```python
from build123d import *

# Parameters (mm, degrees)
SKETCH1_R               = 35
BOSS_EXTRUDE1_DEPTH     = 25
SKETCH2_R               = 30
CUT_EXTRUDE1_DEPTH      = 20
SKETCH3_R               = 25
CUT_EXTRUDE2_DEPTH      = 20
SKETCH4_R               = 27
CUT_EXTRUDE3_DEPTH      = 2.5
SKETCH5_R               = 55.910187051
CUT_EXTRUDE4_DEPTH      = 10
CUT_EXTRUDE6_DEPTH      = 52.720402164
CUT_EXTRUDE6_DEPTH_BACK = 52.720402164
SKETCH7_R               = 3.175


with BuildPart() as part:
    # Sketch1 → Boss-Extrude1 (new body)
    with BuildSketch(Plane(origin=(0, 0, 0), x_dir=(1, 0, 0), z_dir=(0, 1, 0))):
        with Locations(Location((0, 0, 0), (0, 0, 270))):
            Circle(SKETCH1_R)
    extrude(amount=BOSS_EXTRUDE1_DEPTH)

    # Sketch2 → Cut-Extrude1 (cut)
    with BuildSketch(Plane(origin=(0, 25, 0), x_dir=(1, 0, 0), z_dir=(0, 1, 0))):
        with Locations(Location((0, 0, 0), (0, 0, 270))):
            Circle(SKETCH2_R)
    extrude(amount=-CUT_EXTRUDE1_DEPTH, mode=Mode.SUBTRACT)

    # Sketch3 → Cut-Extrude2 (cut)
    with BuildSketch(Plane.XZ):
        with Locations(Location((0, 0, 0), (0, 0, 270))):
            Circle(SKETCH3_R)
    extrude(amount=-CUT_EXTRUDE2_DEPTH, mode=Mode.SUBTRACT)

    # Sketch4 → Cut-Extrude3 (cut)
    with BuildSketch(Plane(origin=(0, 5, 0), x_dir=(1, 0, 0), z_dir=(0, 1, 0))):
        with Locations(Location((0, 0, 0), (0, 0, 270))):
            Circle(SKETCH4_R)
    extrude(amount=-CUT_EXTRUDE3_DEPTH, mode=Mode.SUBTRACT)

    # Sketch5 → Cut-Extrude4 (cut)
    with BuildSketch(Plane(origin=(0, 25, 0), x_dir=(1, 0, 0), z_dir=(0, 1, 0))):
        Circle(SKETCH5_R)
    extrude(amount=-CUT_EXTRUDE4_DEPTH, mode=Mode.SUBTRACT)

    # Sketch7 → Cut-Extrude6 (cut, two sides: drawn at the far end of the back side and taken through both)
    with BuildSketch(Plane.XY.offset(-CUT_EXTRUDE6_DEPTH_BACK)):
        with Locations((0, 9.572)):
            Circle(SKETCH7_R)
    extrude(amount=CUT_EXTRUDE6_DEPTH + CUT_EXTRUDE6_DEPTH_BACK, mode=Mode.SUBTRACT)


solid = part.part
```
Input: part model. Units: mm. Frame: model coordinates. A direction names the side the tool comes from. Give positions to 0.01 mm unless a question says otherwise; leave off trailing zeros. Loops run counter-clockwise (first coordinate to the right, second up) from the corner with the lowest first, then second, coordinate; pieces in that order, holes last.
1) Section query D-D on x = -12.5. Return the cut outline in (y, z).
A:
outline: (0, -32.69) - (15, -32.69) - (15, -27.27) - (5, -27.27) - (5, -23.93) - (2.5, -23.93) - (2.5, -21.65) - (0, -21.65) - close; (0, 21.65) - (2.5, 21.65) - (2.5, 23.93) - (5, 23.93) - (5, 27.27) - (15, 27.27) - (15, 32.69) - (0, 32.69) - close
2) Section query B-B on z = 3.5. Return the cut outline in (x, y), and give its area (3 significant figures).
A:
outline: (-34.82, 0) - (-24.75, 0) - (-24.75, 2.5) - (-26.77, 2.5) - (-26.77, 5) - (-29.8, 5) - (-29.8, 15) - (-34.82, 15) - close; (24.75, 0) - (34.82, 0) - (34.82, 15) - (29.8, 15) - (29.8, 5) - (26.77, 5) - (26.77, 2.5) - (24.75, 2.5) - close
area: 191 mm2
3) Mould query, pull axis X, two halves, no side actions, for faces 3 (the cylindrical face through (-0.688, 6.473, -32.453)), 4 (the flat face through (11, 5, -25)), 5 (the flat face through (26, 15, -16)), 6 (the cylindrical face through (10.513, 7.395, 33.384)). Classes: released by +X, released by -X, zero draft, split by the parting line, or undercut.
A:
face 3: undercut
face 4: undercut
face 5: zero draft
face 6: split by the parting line
4) Contact query for flat-ended pins moving along their axis: pin 1 (3 mm diameter, centred on y = 13, z = 4, fed in from -X); pin 2 (1.5 mm diameter, centred on y = 4.5, z = 8, fed in from -X); pin 3 (18 mm diameter, centred on x = -10.5, z = 10.5, fed in from +Y); pin 4 (1.5 mm diameter, centred on y = 3.5, z = -21, fed in from -X). Output: stop coordinate, or through.
A:
pin 1: stops at x = -34.91
pin 2: stops at x = -34.24
pin 3: passes through
pin 4: stops at x = -28.55
5) Section query A-A on x = 0. Return the cut outline in (y, z).
A:
outline: (0, -35) - (6.4, -35) - (6.4, -30) - (5, -30) - (5, -27) - (2.5, -27) - (2.5, -25) - (0, -25) - close; (0, 25) - (2.5, 25) - (2.5, 27) - (5, 27) - (5, 30) - (6.4, 30) - (6.4, 35) - (0, 35) - close; (12.75, -35) - (15, -35) - (15, -30) - (12.75, -30) - close; (12.75, 30) - (15, 30) - (15, 35) - (12.75, 35) - close
6) Section query C-C on y = 11.25. Return the cut outline in (x, z).
A:
outline: (-2.7, -34.9) - (-2.7, -29.88) arc R30 cw to (-2.7, 29.88) - (-2.7, 34.9) arc R35 ccw to start; (2.7, -34.9) arc R35 ccw to (2.7, 34.9) - (2.7, 29.88) arc R30 cw to (2.7, -29.88) - close
7) Reachability of faces 1 (the flat face through (8, 0, -24)), 2 (the cylindrical face through (-11.49, 10.07, 27.712)) from +Z, -Z, +X, -X, +Y, -Y: full face, straight path, thin tool, end or side. Return the list, or none.
A:
face 1: +Z, -Z, +X, -X, -Y
face 2: +Y
8) Line query: L1, parallel to X at y = 6.25, z = 0; L2, parallel to X at y = 1.6, z = 0; L3, parallel to Y at x = 0, z = -33. Output: solid intervals per line, ascending.
A:
L1: x = -35 to -30, 30 to 35
L2: x = -35 to -25, 25 to 35
L3: y = 0 to 6.4, 12.75 to 15
